```python
from build123d import *

# Parameters (mm, degrees)
EXTRUDE1_DEPTH          = 5.5
SKETCH2_R               = 1.5
SKETCH2_R_2             = 1
CUT_EXTRUDE1_DEPTH      = 19.5
CUT_EXTRUDE1_DEPTH_BACK = 19.5


with BuildPart() as part:
    # Sketch1 → Extrude1 (new body, symmetric)
    with BuildSketch(Plane.XY):
        with BuildLine():
            Line((-40, 18.5), (-30, 18.5))
            Line((-30, 18.5), (-85, 4))
            Line((-85, 4), (-85.527864045, 4))
            ThreePointArc((-85.527864045, 4), (-96, 0), (-85.527864045, -4))
            Line((-85.527864045, -4), (-85, -4))
            Line((-85, -4), (-30, -18.5))
            Line((-30, -18.5), (-40, -18.5))
            ThreePointArc((-40, -18.5), (-102.498734411, -16.871356549), (-164.827821897, -11.989846995))
            Line((-164.827821897, -11.989846995), (-246, -3.5))
            Line((-246, -3.5), (-246, 3.5))
            Line((-246, 3.5), (-164.827821897, 11.989846995))
            ThreePointArc((-164.827821897, 11.989846995), (-102.498734411, 16.871356549), (-40, 18.5))
        make_face()
    extrude(amount=EXTRUDE1_DEPTH, both=True)

    # Sketch2 → Cut-Extrude1 (cut, two sides)
    with BuildSketch(Plane(origin=(0, 0, 0), x_dir=(1, 0, 0), z_dir=(0, 1, 0))) as cut_extrude1_sk:
        with Locations(Location((-63, 0, 0), (0, 0, 270))):  # turned: the seam where the file's is
            Circle(SKETCH2_R)
        with Locations(Location((-78, 0, 0), (0, 0, 270))):  # turned: the seam where the file's is
            Circle(SKETCH2_R_2)
    extrude(amount=CUT_EXTRUDE1_DEPTH, mode=Mode.SUBTRACT)
    extrude(cut_extrude1_sk.sketch, amount=-CUT_EXTRUDE1_DEPTH_BACK, mode=Mode.SUBTRACT)


solid = part.part
```
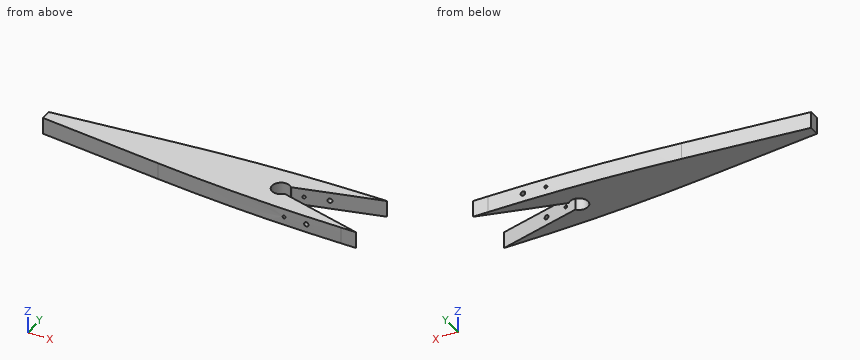
Geometry check sheet. Reference: the model listing, model coordinates, mm. Give positions to 0.01 mm unless a question says otherwise; leave off trailing zeros. Order: outer loops, then holes, each group sorted by start corner. A loop starts at its lowest first (then second) coordinate and runs counter-clockwise, first axis right, second up.
1. Section check B-B, the plane y = 0. Enter the section's corners in (x, z).
2. Gauge pin test, flat ends, axial feed: pin 1 Ø4 at (x, z) = (-63, 0) entering from -Y; pin 2 Ø6 at (x, z) = (-80.5, 0.5) entering from -Y; pin 3 Ø3 at (x, z) = (-64, 4.5) entering from +Y. Record the tip position at first contact, or that the pin passes through.
3. Thickness scan on L1, parallel to Z at x = -63, y = -12.5; L2, parallel to X at y = 0, z = 3; L3, parallel to Y at x = -90, z = 2.5. Record the ranges inside material, lowest first.
4. Section check A-A, the plane x = -90. Enter the section's corners in (y, z).
5. Section check C-C, the plane x = -177. Enter the section's corners in (y, z).
Values follow:
1. outline: (-246, -5.5) - (-96, -5.5) - (-96, 5.5) - (-246, 5.5) - close
2. pin 1: stops at y = -18.32
2. pin 2: stops at y = -17.91
2. pin 3: stops at y = 18.29
3. L1: z = -5.5 to -1.5, 1.5 to 5.5
3. L2: x = -246 to -96
3. L3: y = -17.46 to -6, 6 to 17.46
4. outline: (-17.46, -5.5) - (-6, -5.5) - (-6, 5.5) - (-17.46, 5.5) - close; (6, -5.5) - (17.46, -5.5) - (17.46, 5.5) - (6, 5.5) - close
5. outline: (-10.72, -5.5) - (10.72, -5.5) - (10.72, 5.5) - (-10.72, 5.5) - close
